Part model, mm, in its own coordinate system. A direction names the side the tool comes from. Coordinates: 2 decimals unless noted, no trailing zeros. Order: outer loops, then holes, each group sorted by start corner. A loop starts at its lowest first (then second) coordinate and runs counter-clockwise, first axis right, second up.
from build123d import *

# Parameters (mm, degrees)
BOSS_EXTRUDE1_DEPTH = 4.7625
CHAMFER1_SIZE       = 0.458146619
CHAMFER1_SIZE_2     = 0.508


with BuildPart() as part:
    # Sketch1 → Boss-Extrude1 (new body)
    with BuildSketch(Plane(origin=(0, 0, 0), x_dir=(1, 0, 0), z_dir=(0, 1, 0))):
        with BuildLine():
            ThreePointArc((-39.484622628, 42.989372509), (-38.273971566, 22.097487787), (-56.9722, 12.7))
            Line((-56.9722, 12.7), (-56.9722, 5.950469261))
            ThreePointArc((-56.9722, 5.950469261), (-51.196875, 0), (-56.9722, -5.950469261))
            Line((-56.9722, -5.950469261), (-56.9722, -12.7))
            ThreePointArc((-56.9722, -12.7), (-38.273971566, -22.097487787), (-39.484622628, -42.989372509))
            Line((-39.484622628, -42.989372509), (-33.639357544, -46.364137879))
            ThreePointArc((-33.639357544, -46.364137879), (-25.5984375, -44.337794344), (-23.332842456, -52.31460714))
            Line((-23.332842456, -52.31460714), (-17.487577372, -55.689372509))
            ThreePointArc((-17.487577372, -55.689372509), (0, -44.194975573), (17.487577372, -55.689372509))
            Line((17.487577372, -55.689372509), (23.332842456, -52.31460714))
            ThreePointArc((23.332842456, -52.31460714), (25.5984375, -44.337794344), (33.639357544, -46.364137879))
            Line((33.639357544, -46.364137879), (39.484622628, -42.989372509))
            ThreePointArc((39.484622628, -42.989372509), (38.273971566, -22.097487787), (56.9722, -12.7))
            Line((56.9722, -12.7), (56.9722, -5.950469261))
            ThreePointArc((56.9722, -5.950469261), (51.196875, 0), (56.9722, 5.950469261))
            Line((56.9722, 5.950469261), (56.9722, 12.7))
            ThreePointArc((56.9722, 12.7), (38.273971566, 22.097487787), (39.484622628, 42.989372509))
            Line((39.484622628, 42.989372509), (33.639357544, 46.364137879))
            ThreePointArc((33.639357544, 46.364137879), (25.5984375, 44.337794344), (23.332842456, 52.31460714))
            Line((23.332842456, 52.31460714), (17.487577372, 55.689372509))
            ThreePointArc((17.487577372, 55.689372509), (0, 44.194975573), (-17.487577372, 55.689372509))
            Line((-17.487577372, 55.689372509), (-23.332842456, 52.31460714))
            ThreePointArc((-23.332842456, 52.31460714), (-25.5984375, 44.337794344), (-33.639357544, 46.364137879))
            Line((-33.639357544, 46.364137879), (-39.484622628, 42.989372509))
        make_face()
        with BuildLine():
            Line((1.374815329, 20.455395717), (17.027484671, 11.418322859))
            ThreePointArc((17.027484671, 11.418322859), (18.813175234, 12.157980108), (19.9898, 10.624572859))
            ThreePointArc((19.9898, 10.624572859), (19.524832015, 9.502040844), (18.4023, 9.037072859))
            Line((18.4023, 9.037072859), (18.4023, -9.037072859))
            ThreePointArc((18.4023, -9.037072859), (19.524832015, -9.502040844), (19.9898, -10.624572859))
            ThreePointArc((19.9898, -10.624572859), (18.813175234, -12.157980108), (17.027484671, -11.418322859))
            Line((17.027484671, -11.418322859), (1.374815329, -20.455395717))
            ThreePointArc((1.374815329, -20.455395717), (1.533407249, -20.838270483), (1.5875, -21.249145717))
            ThreePointArc((1.5875, -21.249145717), (-0.410875234, -22.782552967), (-1.374815329, -20.455395717))
            Line((-1.374815329, -20.455395717), (-17.027484671, -11.418322859))
            ThreePointArc((-17.027484671, -11.418322859), (-19.777115329, -11.418322859), (-18.4023, -9.037072859))
            Line((-18.4023, -9.037072859), (-18.4023, 9.037072859))
            ThreePointArc((-18.4023, 9.037072859), (-19.777115329, 11.418322859), (-17.027484671, 11.418322859))
            Line((-17.027484671, 11.418322859), (-1.374815329, 20.455395717))
            ThreePointArc((-1.374815329, 20.455395717), (-0.410875234, 22.782552967), (1.5875, 21.249145717))
            ThreePointArc((1.5875, 21.249145717), (1.533407249, 20.838270483), (1.374815329, 20.455395717))
        make_face(mode=Mode.SUBTRACT)
    extrude(amount=BOSS_EXTRUDE1_DEPTH)

    # Chamfer1
    # the kernel refuses this chamfer: 0.508, 0.458146619 mm, written as the material it takes off along each edge
    with BuildSketch(Plane(origin=(-39.484622628, -1.324398774, 42.989372509), x_dir=(0.8660254037844506, 0, 0.49999999999997935), z_dir=(0, 1, 0)), Plane(origin=(-56.9722, -1.324398774, -12.7), x_dir=(0, 0, 1), z_dir=(0, 1, 0)), Plane(origin=(-17.487577372, -1.324398774, -55.689372509), x_dir=(-0.8660254037844313, 0, 0.5000000000000127), z_dir=(0, 1, 0)), Plane(origin=(39.484622628, -1.324398774, -42.989372509), x_dir=(-0.86602540378444, 0, -0.4999999999999977), z_dir=(0, 1, 0)), Plane(origin=(56.9722, -1.324398774, 12.7), x_dir=(0, 0, -1), z_dir=(0, 1, 0)), Plane(origin=(17.487577372, -1.324398774, 55.689372509), x_dir=(0.8660254037844486, 0, -0.4999999999999827), z_dir=(0, 1, 0))) as chamfer1_piece_1:
        with BuildLine():
            Line((CHAMFER1_SIZE, 0), (0.052567717, 0.512318712))
            ThreePointArc((0.052567717, 0.512318712), (0.028757334, 0.263227837), (0, 0))
            Line((0, 0), (CHAMFER1_SIZE, 0))
        make_face()
    extrude(amount=7.411297548, mode=Mode.SUBTRACT)
    with BuildSketch(Plane(origin=(-56.9722, -1.306414958, 12.7), x_dir=(0.9946357789180702, 0, -0.10343919613011188), z_dir=(0, 1, 0)), Plane(origin=(-39.484622628, -1.306414958, -42.989372509), x_dir=(0.5868988610547448, 0, 0.8096602539909213), z_dir=(0, 1, 0)), Plane(origin=(56.9722, -1.306414958, -12.7), x_dir=(-0.9946357789180716, 0, 0.1034391961300989), z_dir=(0, 1, 0)), Plane(origin=(39.484622628, -1.306414958, 42.989372509), x_dir=(-0.5868988610547374, 0, -0.8096602539909268), z_dir=(0, 1, 0)), Plane(origin=(-17.487577372, -1.306414958, 55.689372509), x_dir=(0.40773691786333366, 0, -0.91309945012102), z_dir=(0, 1, 0))) as chamfer1_piece_2:
        with BuildLine():
            Line((0.462627791, 0), (CHAMFER1_SIZE_2 * 0.10343919613, CHAMFER1_SIZE_2 * 0.994635778918))
            Line((CHAMFER1_SIZE_2 * 0.10343919613, CHAMFER1_SIZE_2 * 0.994635778918), (0, 0))
            ThreePointArc((0, 0), (0.237719559, 0.001403335), (0.462627791, 0))
        make_face()
    extrude(amount=7.375329916, mode=Mode.SUBTRACT)
    with BuildSketch(Plane(origin=(17.487577372, -1.306414958, -55.689372509), x_dir=(0.8660254037844403, 0, 0.49999999999999717), z_dir=(0, 1, 0))) as chamfer1_piece_3:
        with BuildLine():
            Line((CHAMFER1_SIZE_2, 0), (0.047853847, -0.460146153))
            ThreePointArc((0.047853847, -0.460146153), (0.025985327, -0.236299219), (0, 0))
            Line((0, 0), (CHAMFER1_SIZE_2, 0))
        make_face()
    extrude(amount=7.375329916, mode=Mode.SUBTRACT)


solid = part.part
Q1. Cut at B-B on x = 0. Write the cut outline in (y, z).
Results list:
outline: (0, -44.19) - (4.76, -44.19) - (4.76, -22.84) - (0, -22.84) - close; (0, 22.84) - (4.76, 22.84) - (4.76, 44.19) - (0, 44.19) - close
Q2. Cut at C-C on x = 28.5. Write the cut outline in (y, z), and give its area (3 significant figures).
Results list:
outline: (0, -43.54) - (4.76, -43.54) - (4.76, 43.54) - (0, 43.54) - close
area: 415 mm2
Q3. Wall check: line 1 along X through (y, z) = (2, -0.5); line 2 along X through (y, z) = (2.95, -12); line 3 along X through (y, z) = (2, -22). Give the ranges that are in metal, low to high.
Results list:
line 1: x = -51.22 to -18.4, 18.4 to 51.22
line 2: x = -56.97 to -19.19, -17.61 to -16.02, 16.02 to 17.61, 19.19 to 56.97
line 3: x = -38.33 to -1.4, 1.4 to 38.33
Q4. Mould opens along Z. For faces 3 (the face through (-20.57, 2.35, -53.91)), 4 (the face through (56.972, 2, 9)), 5 (the face through (-38.112, 2.348, -22.384)) say: pulls with the +Z half, pulls with the -Z half, needs draft (parallel to the pull), parting line crosses it, or undercut.
Results list:
face 3: pulls with the -Z half
face 4: needs draft
face 5: undercut
Q5. Cut at A-A on z = 0. Write the cut outline in (x, y).
Results list:
outline: (-51.2, 0) - (-18.4, 0) - (-18.4, 4.76) - (-51.2, 4.76) - close; (18.4, 0) - (51.2, 0) - (51.2, 4.76) - (18.4, 4.76) - close
Q6. Which spindle directions (+Z, -Z, +X, -X, +Y, -Y) get a long thin tool onto all of the face, cutting with end or side? Do faces 1 (the face through (-9.09, 2.35, 16)), 2 (the face through (36, 2, 45)). Say none if no direction does.
Results list:
face 1: +Y, -Y
face 2: +Z, +X, +Y, -Y
Q7. Cut at D-D on z = 31. Write the cut outline in (x, y), and give its area (3 significant figures).
Results list:
outline: (-35.73, 0) - (35.73, 0) - (35.73, 4.76) - (-35.73, 4.76) - close
area: 340 mm2
Q8. Pin check, flat tips, straight feed: pin 1 Ø1 at (y, z) = (2, -40) entering from +X; pin 2 Ø3 at (x, z) = (0, -21.25) entering from -Y; pin 3 Ø1.4 at (y, z) = (3, -0.5) entering from -X; pin 4 Ø2 at (x, y) = (-15.5, 1) entering from -Z. Stop position of each tip, or through.
Results list:
pin 1: stops at x = 37.92
pin 2: passes through
pin 3: stops at x = -51.32
pin 4: stops at z = -53.72
